Verification items for the finished model (mm, model axes). Face numbers are marked on the shaded views. A direction names the side the tool comes from. Coordinates: 2 decimals unless noted, no trailing zeros. Write each loop counter-clockwise with the first axis right and the second up, starting at its lowest first coordinate (ties: lowest second). Pieces come first, ordered by that corner, then holes. Notation, with made-up numbers: (68.25, -39.5) - (82.25, -39.5) arc R33 ccw to (82.25, -7.5) - close; hole circle Ø9 at (36.5, -7). An arc over 180 degrees is marked (long way). Use CSV: the item, a comma, the result in double quotes. Start each with the question number.
```python
from build123d import *

# Parameters (mm, degrees)
SKETCH1_W               = 30
SKETCH1_H               = 20
BOSS_EXTRUDE1_DEPTH     = 4
SKETCH2_W               = 30
SKETCH2_H               = 4
BOSS_EXTRUDE2_DEPTH     = 15
CUT_EXTRUDE1_DEPTH      = 2.5
SKETCH4_R               = 1.5
CUT_EXTRUDE2_DEPTH      = 19.5
CUT_EXTRUDE2_DEPTH_BACK = 2.5
CUT_EXTRUDE3_DEPTH      = 16
CUT_EXTRUDE3_DEPTH_BACK = 2.5
SKETCH6_R               = 1.5
CUT_EXTRUDE4_DEPTH      = 18.5
CUT_EXTRUDE4_DEPTH_BACK = 2.5


with BuildPart() as part:
    # Sketch1 → Boss-Extrude1 (new body)
    with BuildSketch(Plane(origin=(0, 0, 0), x_dir=(1, 0, 0), z_dir=(0, 1, 0))):
        Rectangle(SKETCH1_W, SKETCH1_H)
    extrude(amount=BOSS_EXTRUDE1_DEPTH)

    # Sketch2 → Boss-Extrude2 (add)
    with BuildSketch(Plane(origin=(0, 4, 0), x_dir=(1, 0, 0), z_dir=(0, 1, 0))):
        with Locations((0, 8)):
            Rectangle(SKETCH2_W, SKETCH2_H)
    extrude(amount=BOSS_EXTRUDE2_DEPTH)

    # Sketch3 → Cut-Extrude1 (cut)
    with BuildSketch(Plane.XY.offset(-6)):
        Polygon((-8.438267522, 12.016236672), (-6.876535044, 14.721236672), (-8.438267522, 17.426236672), (-11.561732478, 17.426236672), (-13.123464956, 14.721236672), (-11.561732478, 12.016236672), align=None)
        Polygon((1.573279484, 11.993045001), (3.146558967, 14.718045001), (1.573279484, 17.443045001), (-1.573279484, 17.443045001), (-3.146558967, 14.718045001), (-1.573279484, 11.993045001), align=None)
        Polygon((12.46124414, 11.971236672), (14.048957381, 14.721236672), (12.46124414, 17.471236672), (9.28581766, 17.471236672), (7.69810442, 14.721236672), (9.28581766, 11.971236672), align=None)
        Polygon((-4.147076238, 5.256448413), (-2.544929241, 8.031448413), (-4.147076238, 10.806448413), (-7.351370232, 10.806448413), (-8.953517229, 8.031448413), (-7.351370232, 5.256448413), align=None)
        Polygon((7.240820874, 5.231448413), (8.857401628, 8.031448413), (7.240820874, 10.831448413), (4.007659367, 10.831448413), (2.391078613, 8.031448413), (4.007659367, 5.231448413), align=None)
    extrude(amount=-CUT_EXTRUDE1_DEPTH, mode=Mode.SUBTRACT)

    # Sketch4 → Cut-Extrude2 (cut, two sides)
    with BuildSketch(Plane.XY.offset(-8.5)) as cut_extrude2_sk:
        with Locations((-10, 14.721236672)):
            Circle(SKETCH4_R)
        with Locations((0, 14.718045001)):
            Circle(SKETCH4_R)
        with Locations((10.8735309, 14.721236672)):
            Circle(SKETCH4_R)
        with Locations((5.624240121, 8.031448413)):
            Circle(SKETCH4_R)
        with Locations((-5.749223235, 8.031448413)):
            Circle(SKETCH4_R)
    extrude(amount=CUT_EXTRUDE2_DEPTH, mode=Mode.SUBTRACT)
    extrude(cut_extrude2_sk.sketch, amount=-CUT_EXTRUDE2_DEPTH_BACK, mode=Mode.SUBTRACT)

    # Sketch5 → Cut-Extrude3 (cut, two sides)
    with BuildSketch(Plane(origin=(0, 4, 0), x_dir=(1, 0, 0), z_dir=(0, 1, 0))) as cut_extrude3_sk:
        Polygon((-9.874222434, -1.236448413), (-8.312489956, 1.468551587), (-9.874222434, 4.173551587), (-12.99768739, 4.173551587), (-14.559419869, 1.468551587), (-12.99768739, -1.236448413), align=None)
        Polygon((-0.207729888, -1.256448413), (1.365549596, 1.468551587), (-0.207729888, 4.193551587), (-3.354288855, 4.193551587), (-4.927568339, 1.468551587), (-3.354288855, -1.256448413), align=None)
        Polygon((9.524140966, -1.281448413), (11.111854207, 1.468551587), (9.524140966, 4.218551587), (6.348714486, 4.218551587), (4.761001245, 1.468551587), (6.348714486, -1.281448413), align=None)
        Polygon((-5.365661597, -8.118028115), (-3.7635146, -5.343028115), (-5.365661597, -2.568028115), (-8.569955591, -2.568028115), (-10.172102588, -5.343028115), (-8.569955591, -8.118028115), align=None)
        Polygon((5.178599497, -7.955553444), (6.795180251, -5.155553444), (5.178599497, -2.355553444), (1.945437989, -2.355553444), (0.328857236, -5.155553444), (1.945437989, -7.955553444), align=None)
    extrude(amount=CUT_EXTRUDE3_DEPTH, mode=Mode.SUBTRACT)
    extrude(cut_extrude3_sk.sketch, amount=-CUT_EXTRUDE3_DEPTH_BACK, mode=Mode.SUBTRACT)

    # Sketch6 → Cut-Extrude4 (cut, two sides)
    with BuildSketch(Plane(origin=(0, 1.5, 0), x_dir=(1, 0, 0), z_dir=(0, 1, 0))) as cut_extrude4_sk:
        with Locations((-11.435954912, 1.468551587)):
            Circle(SKETCH6_R)
        with Locations((-1.781009372, 1.468551587)):
            Circle(SKETCH6_R)
        with Locations((7.936427726, 1.468551587)):
            Circle(SKETCH6_R)
        with Locations((3.562018743, -5.155553444)):
            Circle(SKETCH6_R)
        with Locations((-6.967808594, -5.343028115)):
            Circle(SKETCH6_R)
    extrude(amount=CUT_EXTRUDE4_DEPTH, mode=Mode.SUBTRACT)
    extrude(cut_extrude4_sk.sketch, amount=-CUT_EXTRUDE4_DEPTH_BACK, mode=Mode.SUBTRACT)


solid = part.part
```
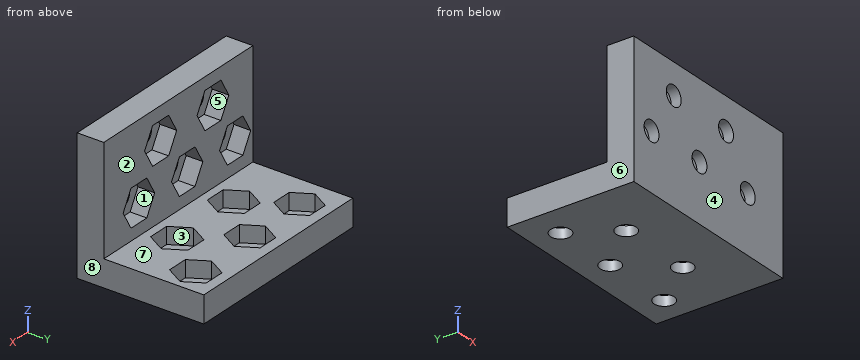
Q1. Scan lines: line 1 along X through (y, z) = (7.25, -9); line 2 along X through (y, z) = (10.75, -8.25); line 3 along Y through (x, z) = (4.5, -7.75). Record each from-to range of solid material in increasing order. Write a range as from..to.
Q2. Gauge pin test, flat ends, axial feed: pin 1 (4 mm diameter, centred on x = -1.78, z = -1.47, fed in from +Y); pin 2 (1.8 mm diameter, centred on x = 0, y = 14.72, fed in from +Z); pin 3 (6 mm diameter, centred on x = -12, z = -1, fed in from +Y); pin 4 (4 mm diameter, centred on x = 10.87, y = 14.72, fed in from +Z). Record the tip position at first contact, or that the pin passes through.
Q3. Tool access check on the marked faces 1, 2, 3 and 4. Record the directions out of +Z, -Z, +X, -X, +Y, -Y that give a thin tool (end or side, any length) a straight path to the whole face; none if there is none.
Q4. Cross-section at B-B (y = 3). State how many separate pieces and enclosed holes the cut face has, plus the area to 3 significant figures.
Q5. Release check for a two-part mould opening along X. For the marked faces 5, 6, 7 and 8 record: released by +X, released by -X, zero draft, split by the parting line, or undercut.
Q6. Cross-section at A-A (y = 7.5). Record the cut outline in (x, z), plus the area to 3 significant figures.
Q7. Cross-section at C-C (z = -4.75). Record the cut outline in (x, y).
Reply:
1,line 1,"-15..-7.03, -4.47..4.34, 6.9..15"
1,line 2,"-15..-7.38, -4.11..3.96, 7.29..15"
1,line 3,"0..5.23, 10.83..19"
2,pin 1,"y = 1.5"
2,pin 2,"through"
2,pin 3,"y = 4"
2,pin 4,"z = -8.5"
3,face 1,"+Y"
3,face 2,"+Z, +X, -X, +Y"
3,face 3,"+Z"
3,face 4,"+Z, -Z, +X, -X, -Y"
4,separate pieces,"1"
4,enclosed holes,"5"
4,area,"469 mm^2"
5,face 5,"undercut"
5,face 6,"released by -X"
5,face 7,"zero draft"
5,face 8,"released by +X"
6,outline,"(-15, -10) - (-7.15, -10) - (-7.15, -8.5) - (-8.65, -8.5) - (-8.65, -6) - (-15, -6) - close; (-4.35, -10) - (4.22, -10) - (4.22, -8.5) - (2.7, -8.5) - (2.7, -6) - (-2.85, -6) - (-2.85, -8.5) - (-4.35, -8.5) - close; (7.03, -10) - (15, -10) - (15, -6) - (8.55, -6) - (8.55, -8.5) - (7.03, -8.5) - close"
6,area,"82.5 mm^2"
7,outline,"(-15, 0) - (15, 0) - (15, 4) - (-15, 4) - close"
